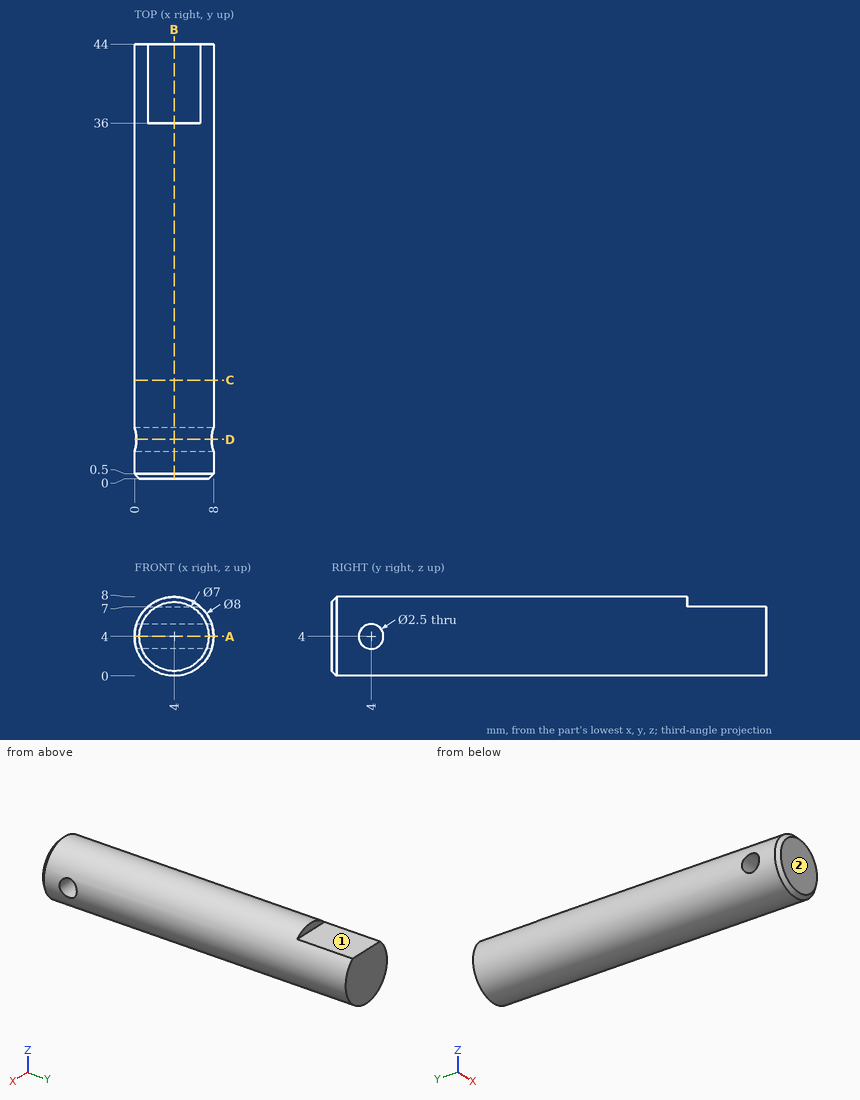
Check sheet for the drawn part. Datum: minimum x, y, z corner. Units: mm. A direction names the side the tool comes from. Coordinates: 2 decimals unless noted, no trailing zeros. Write each loop counter-clockwise with the first axis right and the second up, starting at its lowest first coordinate (ties: lowest second). Pieces come first, ordered by that corner, then holes. Notation, with made-up numbers: M 62.25,-27.5 L 73.25,-27.5 A9 ccw 73.25,-13.5 Z; hole C 1,78 d1. An arc over 180 degrees is marked long. One line per item, written item: value.
Item 1: Section check D-D, the plane y = 4. Record the boundary of the cut face in (x, z).
Check sheet entries:
outline: M 0.2,2.75 A4 ccw 7.8,2.75 Z; M 0.2,5.25 L 7.8,5.25 A4 ccw Z
Item 2: Section check A-A, the plane z = 4. Record the boundary of the cut face in (x, y).
Check sheet entries:
outline: M 0,0.5 L 0.5,0 L 7.5,0 L 8,0.5 L 8,2.75 L 0,2.75 Z; M 0,5.25 L 8,5.25 L 8,44 L 0,44 Z
Item 3: Scan lines: line 1 along Z through (x, y) = (4.25, 4); line 2 along X through (y, z) = (33, 3.75); line 3 along Z through (x, y) = (4.75, 4). Record each from-to range of solid material in increasing order.
Check sheet entries:
line 1: z = 0.01 to 2.75, 5.25 to 7.99
line 2: x = 0.01 to 7.99
line 3: z = 0.07 to 2.75, 5.25 to 7.93
Item 4: Section check B-B, the plane x = 4. Record the boundary of the cut face in (y, z), plus the area to 3 significant figures.
Check sheet entries:
outline: M 0,0.5 L 0.5,0 L 44,0 L 44,7 L 36,7 L 36,8 L 0.5,8 L 0,7.5 Z; hole C 4,4 d2.5
area: 339 mm^2
Item 5: Access from +Z, -Z, +X, -X, +Y, -Y to the whole of each face (thin tool, end or side, straight path). Record for the marked faces 1 and 2.
Check sheet entries:
face 1: +Z, +X, -X, +Y
face 2: +Z, -Z, +X, -X, -Y
Item 6: Gauge pin test, flat ends, axial feed: pin 1 Ø0.5 at (x, z) = (4.5, 7.5) entering from +Y; pin 2 Ø4 at (y, z) = (26, 6.5) entering from -X; pin 3 Ø4 at (x, y) = (1, 16.5) entering from -Z. Record the tip position at first contact, or that the pin passes through.
Check sheet entries:
pin 1: stops at y = 36
pin 2: stops at x = 0.03
pin 3: stops at z = 0.13
Item 7: Section check C-C, the plane y = 10. Record the boundary of the cut face in (x, z), plus the area to 3 significant figures.
Check sheet entries:
outline: C 4,4 d8
area: 50.3 mm^2
